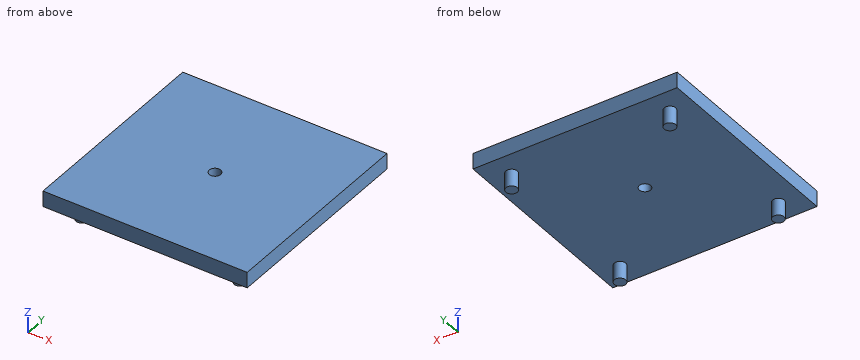
from build123d import *

# Parameters (mm, degrees)
SKETCH1_W           = 113.157
SKETCH1_H           = 113.157
SKETCH1_R           = 3.175
SKETCH1_R_2         = 51.59375
BOSS_EXTRUDE1_DEPTH = 8.73125
SKETCH1_5_R         = 3.175
BOSS_EXTRUDE4_DEPTH = 9.398


with BuildPart() as part:
    # Sketch1 → Boss-Extrude1 (new body)
    with BuildSketch(Plane.XY):
        Rectangle(SKETCH1_W, SKETCH1_H)
        with Locations((-43.8785, -43.8785)):
            Circle(SKETCH1_R, mode=Mode.SUBTRACT)
        with Locations((43.8785, -43.8785)):
            Circle(SKETCH1_R, mode=Mode.SUBTRACT)
        with Locations((43.8785, 43.8785)):
            Circle(SKETCH1_R, mode=Mode.SUBTRACT)
        with Locations((-43.8785, 43.8785)):
            Circle(SKETCH1_R, mode=Mode.SUBTRACT)
        Circle(SKETCH1_R_2, mode=Mode.SUBTRACT)
        with Locations((43.8785, 43.8785)):
            Circle(SKETCH1_R)
        with Locations((-43.8785, 43.8785)):
            Circle(SKETCH1_R)
        with Locations((-43.8785, -43.8785)):
            Circle(SKETCH1_R)
        with Locations((43.8785, -43.8785)):
            Circle(SKETCH1_R)
        Circle(SKETCH1_R_2)
        with Locations((41.273292929, 7.277595126)):
            Circle(SKETCH1_R, mode=Mode.SUBTRACT)
        with Locations((-26.939228722, 32.104922611)):
            Circle(SKETCH1_R, mode=Mode.SUBTRACT)
        Circle(SKETCH1_R, mode=Mode.SUBTRACT)
        with Locations((-14.334064207, -39.382517737)):
            Circle(SKETCH1_R, mode=Mode.SUBTRACT)
        with Locations((41.273292929, 7.277595126)):
            Circle(SKETCH1_R)
        with Locations((-26.939228722, 32.104922611)):
            Circle(SKETCH1_R)
        with Locations((-14.334064207, -39.382517737)):
            Circle(SKETCH1_R)
    extrude(amount=BOSS_EXTRUDE1_DEPTH)

    # Sketch1_5 → Boss-Extrude4 (add)
    with BuildSketch(Plane.XY):
        with Locations((43.8785, 43.8785)):
            Circle(SKETCH1_5_R)
        with Locations((-43.8785, 43.8785)):
            Circle(SKETCH1_5_R)
        with Locations((-43.8785, -43.8785)):
            Circle(SKETCH1_5_R)
        with Locations((43.8785, -43.8785)):
            Circle(SKETCH1_5_R)
    extrude(amount=-BOSS_EXTRUDE4_DEPTH)


solid = part.part
Design review of the part built by this model. Coordinates are the model's own, in mm. Coordinates: 2 decimals unless noted, no trailing zeros. Order: outer loops, then holes, each group sorted by start corner. A loop starts at its lowest first (then second) coordinate and runs counter-clockwise, first axis right, second up. Notation, with made-up numbers: (-33.75, 76.5) -> (14.25, 76.5) arc R29 cw to (14.25, 101.5) -> close; hole circle Ø6 at (83, 10.25). An arc over 180 degrees is marked (long way). Use one line per item in the form item = value. Start each with the question number.
(1) Add section C-C on z = -2. Give the number of separate pieces and of enclosed holes in the cut face, plus the area to 3 significant figures.
(2) Add section A-A on y = 0. State the section outline as (x, z) points (1 decimal), plus the area to 3 significant figures.
(3) Add section D-D on y = 39. State the section outline as (x, z) points, plus the area to 3 significant figures.
(4) For probe 1 along Y at (x, z) = (0, 5.75) (1 decimal); probe 2 along Z at (x, y) = (-37, 51.5); probe 3 along X at (y, z) = (1.5, 1.75), list the stretches that pass through material, from the lowest coordinate up.
(5) Insertion check: pin 1 (2 mm diameter, centred on x = 36.5, y = -6, fed in from -Z); pin 2 (10 mm diameter, centred on y = 17, z = -0.5, fed in from -X); pin 3 (10 mm diameter, centred on x = -9, z = -6.5, fed in from -Y). Each pin has a flat end and moves straight along its axis. Give the tip position at first contact, or say it passes through.
Answer block:
q1.separate_pieces = 4
q1.enclosed_holes = 0
q1.area = 127 mm²
q2.outline = (-56.6, 0) -> (-3.2, 0) -> (-3.2, 8.7) -> (-56.6, 8.7) -> close; (3.2, 0) -> (56.6, 0) -> (56.6, 8.7) -> (3.2, 8.7) -> close
q2.area = 933 mm²
q3.outline = (-56.58, 0) -> (56.58, 0) -> (56.58, 8.73) -> (-56.58, 8.73) -> close
q3.area = 988 mm²
q4.probe_1 = -56.6 to -3.2, 3.2 to 56.6
q4.probe_2 = 0 to 8.73
q4.probe_3 = -56.58 to -2.8, 2.8 to 56.58
q5.pin_1 = 0
q5.pin_2 = -56.58
q5.pin_3 = through
